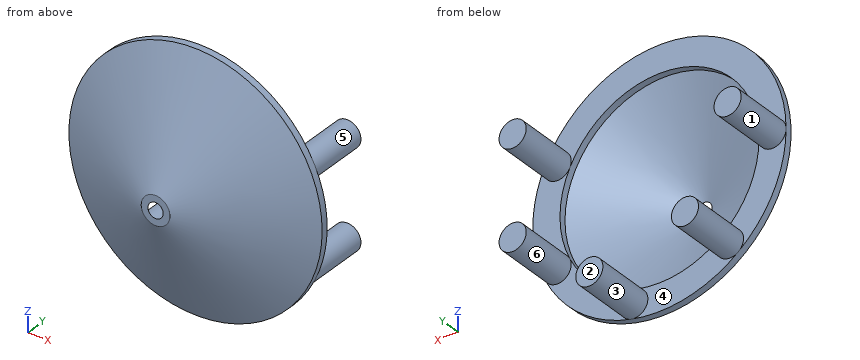
```python
from build123d import *

# Parameters (mm, degrees)
SKETCH3_R           = 3
BOSS_EXTRUDE1_DEPTH = 15
CIRPATTERN1_COUNT   = 5
CIRPATTERN1_ANGLE   = 205.714285714


with BuildPart() as part:
    # Sketch1 → Revolve1 (revolve)
    with BuildSketch(Plane.XY):
        Polygon((28, 0), (3.175, -12), (1.68595, -12), (22, 0), (22, 1.5), (28, 1.5), align=None)
    revolve(axis=Axis((0, -582.446756226, 0), (0, 1, 0)))

    # Sketch3 → Boss-Extrude1 (add)
    with BuildSketch(Plane(origin=(0, 0, 0), x_dir=(1, 0, 0), z_dir=(0, 1, 0))):
        with Locations((-25, 0)):
            Circle(SKETCH3_R)
    boss_extrude1 = extrude(amount=BOSS_EXTRUDE1_DEPTH)

    # CirPattern1: Boss-Extrude1 ×5 about axis
    cirpattern1_axis = Axis((0, 0, 0), (0, -1, 0))
    for i in range(1, CIRPATTERN1_COUNT):
        add(boss_extrude1.rotate(cirpattern1_axis, i * CIRPATTERN1_ANGLE / (CIRPATTERN1_COUNT - 1)))


solid = part.part
```
Work out the finished part from the listing and answer in its coordinate system (mm). Face numbers are marked on the shaded views. A direction names the side the tool comes from. Coordinates: 2 decimals unless noted, no trailing zeros. Loops run counter-clockwise (first coordinate to the right, second up) from the corner with the lowest first, then second, coordinate; pieces in that order, holes last. Notation, with made-up numbers: (19.5, 61.25) - (75.5, 61.25) arc R14 ccw to (75.5, 78.25) - close; hole circle Ø11 at (54, 50.5). An arc over 180 degrees is marked (long way). Use a Markdown table: item, result.
Item 1: The mould has two halves that part along Z. Classify the marked faces 3, 4, 5 and 6: +Z half, -Z half, draft (parallel to the pull), parting line (faces both ways), or undercut.
Evaluation:
| item | result |
|---|---|
| face 3 | parting line |
| face 4 | draft |
| face 5 | undercut |
| face 6 | undercut |
Item 2: Find section B-B, the plane y = 10.5. Determine the outline of the cut face in (x, z), and give its area (3 significant figures).
Evaluation:
| item | result |
|---|---|
| outline | circle Ø6 at (-25, 0); circle Ø6 at (-15.59, -19.55); circle Ø6 at (5.56, -24.37); circle Ø6 at (22.52, -10.85); circle Ø6 at (22.52, 10.85) |
| area | 141 mm2 |
Item 3: Consider probe 1 along X at (y, z) = (0.75, 0); probe 2 along Z at (x, y) = (-3, -0.5). Determine where each line is inside the solid, lowest interval first. Write a range as from..to.
Evaluation:
| item | result |
|---|---|
| probe 1 | x = -28..-22, 22..28 |
| probe 2 | z = -26.8..-20.94, 20.94..26.8 |
Item 4: Find section C-C, the plane y = -5. Determine the outline of the cut face in (x, z), and give its area (3 significant figures).
Evaluation:
| item | result |
|---|---|
| outline | circle Ø35.31 at (0, 0); hole circle Ø27.07 at (0, 0) |
| area | 404 mm2 |
Item 5: Find section D-D, the plane y = -8. Determine the outline of the cut face in (x, z).
Evaluation:
| item | result |
|---|---|
| outline | circle Ø22.9 at (0, 0); hole circle Ø16.91 at (0, 0) |
Item 6: Find section A-A, the plane x = 0. Determine the outline of the cut face in (y, z) (3 decimals), and give its area (3 significant figures).
Evaluation:
| item | result |
|---|---|
| outline | (-12, -3.175) - (0, -28) - (1.5, -28) - (1.5, -22) - (0, -22) - (-12, -1.686) - close; (-12, 1.686) - (0, 22) - (1.5, 22) - (1.5, 28) - (0, 28) - (-12, 3.175) - close |
| area | 108 mm2 |
Item 7: Given pin 1 Ø9 at (x, z) = (15, -18) entering from +Y; pin 2 Ø22.5 at (x, z) = (7.5, 7.5) entering from +Y; pin 3 Ø1 at (x, z) = (6.5, -20) entering from +Y, each flat-ended and moving along its own axis, determine where each tip first touches the part or whether it passes through.
Evaluation:
| item | result |
|---|---|
| pin 1 | stops at y = 1.5 |
| pin 2 | stops at y = -0.08 |
| pin 3 | stops at y = -0.28 |
Item 8: For the marked faces 1 and 2, determine the directions among +Z, -Z, +X, -X, +Y, -Y from which every point of the face is accessible in a straight line to the end or side of a thin tool.
Evaluation:
| item | result |
|---|---|
| face 1 | +Y |
| face 2 | +Z, -Z, +X, -X, +Y |
